Input: part model. Units: mm. Frame: model coordinates. Round coordinates to 2 decimals unless told otherwise and drop trailing zeros. Loops run counter-clockwise (first coordinate to the right, second up) from the corner with the lowest first, then second, coordinate; pieces in that order, holes last.
1) Section C-C, the plane x = -9. Return loops of the section in (y, z), and give its area (3 significant figures).
2) First-contact query: pin 1 (10 mm diameter, centred on x = -5.5, z = 354, fed in from +Y); pin 2 (1.2 mm diameter, centred on y = -1, z = 171.5, fed in from +X); pin 3 (1.2 mm diameter, centred on y = -1, z = 317, fed in from -X). Flat tips, straight axial feed; report the tip coordinate or a pass-through.
3) Ray query, line 1 along X through (y, z) = (-0.25, 343.5); line 2 along X through (y, z) = (4.75, 322.5); line 3 along Y through (x, z) = (-8.5, 91.5). Return the intervals inside material, ascending.
4) Section A-A, the plane z = 383. Return loops of the section in (x, y).
5) Section B-B, the plane y = 2.75. Return loops of the section in (x, z), and give its area (3 significant figures).
6) Draft query along X for faces 1 (the face through (-3, 0, 208)), 2 (the face through (-0.1, -0.3, 410)). Return one class per face: pulls with the +X half, pulls with the -X half, needs draft (parallel to the pull), parting line crosses it, or undercut.
from build123d import *

# Parameters (mm, degrees)
CROQUIS1_W              = 35
CROQUIS1_H              = 410
SALIENTE_EXTRUIR1_DEPTH = 7
CROQUIS2_W              = 25
CROQUIS2_H              = 5.5
CORTAR_EXTRUIR1_DEPTH   = 411
CROQUIS3_W              = 3.5
CROQUIS3_H              = 5.5
CORTAR_EXTRUIR2_DEPTH   = 411
CROQUIS4_W              = 3.5
CROQUIS4_H              = 5.5
CORTAR_EXTRUIR3_DEPTH   = 411
CORTAR_EXTRUIR4_DEPTH   = 2.5
CORTAR_EXTRUIR5_DEPTH   = 2.5
CORTAR_EXTRUIR6_DEPTH   = 2.5
CORTAR_EXTRUIR7_DEPTH   = 2.5
CORTAR_EXTRUIR8_DEPTH   = 2.5
CORTAR_EXTRUIR9_DEPTH   = 2.5
CORTAR_EXTRUIR10_DEPTH  = 2.5
CORTAR_EXTRUIR11_DEPTH  = 2.5
CORTAR_EXTRUIR12_DEPTH  = 2.5
CORTAR_EXTRUIR13_DEPTH  = 2.5
CORTAR_EXTRUIR14_DEPTH  = 8


with BuildPart() as part:
    # Croquis1 → Saliente-Extruir1 (new body)
    with BuildSketch(Plane.XZ.offset(1.5)):
        with Locations((0, 205)):
            Rectangle(CROQUIS1_W, CROQUIS1_H)
    extrude(amount=-SALIENTE_EXTRUIR1_DEPTH)

    # Croquis2 → Cortar-Extruir1 (cut, through all)
    with BuildSketch(Plane.XY.offset(410)):
        with Locations((0, 2.75)):
            Rectangle(CROQUIS2_W, CROQUIS2_H)
    extrude(amount=-CORTAR_EXTRUIR1_DEPTH, mode=Mode.SUBTRACT)

    # Croquis3 → Cortar-Extruir2 (cut, through all)
    with BuildSketch(Plane.XY.offset(410)):
        with Locations((15.75, 1.25)):
            Rectangle(CROQUIS3_W, CROQUIS3_H)
    extrude(amount=-CORTAR_EXTRUIR2_DEPTH, mode=Mode.SUBTRACT)

    # Croquis4 → Cortar-Extruir3 (cut, through all)
    with BuildSketch(Plane.XY.offset(410)):
        with Locations((-15.75, 1.25)):
            Rectangle(CROQUIS4_W, CROQUIS4_H)
    extrude(amount=-CORTAR_EXTRUIR3_DEPTH, mode=Mode.SUBTRACT)

    # Croquis5 → Cortar-Extruir4 (cut, through all)
    with BuildSketch(Plane(origin=(0, 0, 0), x_dir=(-1, 0, 0), z_dir=(0, 1, 0))):
        with BuildLine():
            Line((-2.7, 402.5), (-2.7, 377.5))
            ThreePointArc((-2.7, 377.5), (0, 374.8), (2.7, 377.5))
            Line((2.7, 377.5), (2.7, 402.5))
            ThreePointArc((2.7, 402.5), (0, 405.2), (-2.7, 402.5))
        make_face()
    extrude(amount=-CORTAR_EXTRUIR4_DEPTH, mode=Mode.SUBTRACT)

    # Croquis6 → Cortar-Extruir5 (cut, through all)
    with BuildSketch(Plane(origin=(0, 0, 0), x_dir=(-1, 0, 0), z_dir=(0, 1, 0))):
        with BuildLine():
            Line((-2.7, 365.5), (-2.7, 340.5))
            ThreePointArc((-2.7, 340.5), (0, 337.8), (2.7, 340.5))
            Line((2.7, 340.5), (2.7, 365.5))
            ThreePointArc((2.7, 365.5), (0, 368.2), (-2.7, 365.5))
        make_face()
    extrude(amount=-CORTAR_EXTRUIR5_DEPTH, mode=Mode.SUBTRACT)

    # Croquis7 → Cortar-Extruir6 (cut, through all)
    with BuildSketch(Plane(origin=(0, 0, 0), x_dir=(-1, 0, 0), z_dir=(0, 1, 0))):
        with BuildLine():
            Line((-2.7, 328.5), (-2.7, 303.5))
            ThreePointArc((-2.7, 303.5), (0, 300.8), (2.7, 303.5))
            Line((2.7, 303.5), (2.7, 328.5))
            ThreePointArc((2.7, 328.5), (0, 331.2), (-2.7, 328.5))
        make_face()
    extrude(amount=-CORTAR_EXTRUIR6_DEPTH, mode=Mode.SUBTRACT)

    # Croquis8 → Cortar-Extruir7 (cut, through all)
    with BuildSketch(Plane(origin=(0, 0, 0), x_dir=(-1, 0, 0), z_dir=(0, 1, 0))):
        with BuildLine():
            Line((-2.7, 291.5), (-2.7, 266.5))
            ThreePointArc((-2.7, 266.5), (0, 263.8), (2.7, 266.5))
            Line((2.7, 266.5), (2.7, 291.5))
            ThreePointArc((2.7, 291.5), (0, 294.2), (-2.7, 291.5))
        make_face()
    extrude(amount=-CORTAR_EXTRUIR7_DEPTH, mode=Mode.SUBTRACT)

    # Croquis9 → Cortar-Extruir8 (cut, through all)
    with BuildSketch(Plane(origin=(0, 0, 0), x_dir=(-1, 0, 0), z_dir=(0, 1, 0))):
        with BuildLine():
            Line((-2.7, 254.5), (-2.7, 229.5))
            ThreePointArc((-2.7, 229.5), (0, 226.8), (2.7, 229.5))
            Line((2.7, 229.5), (2.7, 254.5))
            ThreePointArc((2.7, 254.5), (0, 257.2), (-2.7, 254.5))
        make_face()
    extrude(amount=-CORTAR_EXTRUIR8_DEPTH, mode=Mode.SUBTRACT)

    # Croquis10 → Cortar-Extruir9 (cut, through all)
    with BuildSketch(Plane(origin=(0, 0, 0), x_dir=(-1, 0, 0), z_dir=(0, 1, 0))):
        with BuildLine():
            Line((-2.7, 217.5), (-2.7, 192.5))
            ThreePointArc((-2.7, 192.5), (0, 189.8), (2.7, 192.5))
            Line((2.7, 192.5), (2.7, 217.5))
            ThreePointArc((2.7, 217.5), (0, 220.2), (-2.7, 217.5))
        make_face()
    extrude(amount=-CORTAR_EXTRUIR9_DEPTH, mode=Mode.SUBTRACT)

    # Croquis11 → Cortar-Extruir10 (cut, through all)
    with BuildSketch(Plane(origin=(0, 0, 0), x_dir=(-1, 0, 0), z_dir=(0, 1, 0))):
        with BuildLine():
            Line((-2.7, 180.5), (-2.7, 155.5))
            ThreePointArc((-2.7, 155.5), (0, 152.8), (2.7, 155.5))
            Line((2.7, 155.5), (2.7, 180.5))
            ThreePointArc((2.7, 180.5), (0, 183.2), (-2.7, 180.5))
        make_face()
    extrude(amount=-CORTAR_EXTRUIR10_DEPTH, mode=Mode.SUBTRACT)

    # Croquis12 → Cortar-Extruir11 (cut, through all)
    with BuildSketch(Plane(origin=(0, 0, 0), x_dir=(-1, 0, 0), z_dir=(0, 1, 0))):
        with BuildLine():
            Line((-2.7, 143.5), (-2.7, 118.5))
            ThreePointArc((-2.7, 118.5), (0, 115.8), (2.7, 118.5))
            Line((2.7, 118.5), (2.7, 143.5))
            ThreePointArc((2.7, 143.5), (0, 146.2), (-2.7, 143.5))
        make_face()
    extrude(amount=-CORTAR_EXTRUIR11_DEPTH, mode=Mode.SUBTRACT)

    # Croquis13 → Cortar-Extruir12 (cut, through all)
    with BuildSketch(Plane(origin=(0, 0, 0), x_dir=(-1, 0, 0), z_dir=(0, 1, 0))):
        with BuildLine():
            Line((-2.7, 106.5), (-2.7, 81.5))
            ThreePointArc((-2.7, 81.5), (0, 78.8), (2.7, 81.5))
            Line((2.7, 81.5), (2.7, 106.5))
            ThreePointArc((2.7, 106.5), (0, 109.2), (-2.7, 106.5))
        make_face()
    extrude(amount=-CORTAR_EXTRUIR12_DEPTH, mode=Mode.SUBTRACT)

    # Croquis14 → Cortar-Extruir13 (cut, through all)
    with BuildSketch(Plane(origin=(0, 0, 0), x_dir=(-1, 0, 0), z_dir=(0, 1, 0))):
        with BuildLine():
            Line((-2.7, 69.5), (-2.7, 44.5))
            ThreePointArc((-2.7, 44.5), (0, 41.8), (2.7, 44.5))
            Line((2.7, 44.5), (2.7, 69.5))
            ThreePointArc((2.7, 69.5), (0, 72.2), (-2.7, 69.5))
        make_face()
    extrude(amount=-CORTAR_EXTRUIR13_DEPTH, mode=Mode.SUBTRACT)

    # Croquis15 → Cortar-Extruir14 (cut, through all)
    with BuildSketch(Plane.XZ.offset(1.5)):
        with BuildLine():
            Line((-2.7, 32.5), (-2.7, 7.5))
            ThreePointArc((-2.7, 7.5), (0, 4.8), (2.7, 7.5))
            Line((2.7, 7.5), (2.7, 32.5))
            ThreePointArc((2.7, 32.5), (0, 35.2), (-2.7, 32.5))
        make_face()
    extrude(amount=-CORTAR_EXTRUIR14_DEPTH, mode=Mode.SUBTRACT)


solid = part.part
Final values:
1. outline: (-1.5, 0) - (0, 0) - (0, 410) - (-1.5, 410) - close
1. area: 615 mm2
2. pin 1: stops at y = 0
2. pin 2: stops at x = 14
2. pin 3: stops at x = -14
3. line 1: x = -14 to -2.7, 2.7 to 14
3. line 2: x = -17.5 to -12.5, 12.5 to 17.5
3. line 3: y = -1.5 to 0
4. outline: (-17.5, 4) - (-14, 4) - (-14, -1.5) - (-2.7, -1.5) - (-2.7, 0) - (-12.5, 0) - (-12.5, 5.5) - (-17.5, 5.5) - close; (2.7, -1.5) - (14, -1.5) - (14, 4) - (17.5, 4) - (17.5, 5.5) - (12.5, 5.5) - (12.5, 0) - (2.7, 0) - close
5. outline: (-14, 0) - (-12.5, 0) - (-12.5, 410) - (-14, 410) - close; (12.5, 0) - (14, 0) - (14, 410) - (12.5, 410) - close
5. area: 1,230 mm2
6. face 1: undercut
6. face 2: needs draft
